Source: CAD feature listing. Evaluate the final solid. Frame: model axes, mm. A direction names the side the tool comes from. Give positions to 0.01 mm unless a question says otherwise; leave off trailing zeros. Loops run counter-clockwise (first coordinate to the right, second up) from the corner with the lowest first, then second, coordinate; pieces in that order, holes last. Notation, with made-up numbers: (-37.75, 72) - (-30.75, 72) arc R30 ccw to (-30.75, 111) - close; hole circle Ø6 at (-22.5, 48). An arc over 180 degrees is marked (long way). Write each question's results on one line, items separated by ' | '. Start each with the question number.
(1) Cut plane D-D on z = -5. Return the cut outline in (x, y).
(2) Cut plane C-C on x = 12.5. Return the cut outline in (y, z), then the cut area to 3 significant figures.
(3) Material intervals for line 1 along Z through (x, y) = (0, 5.1); line 2 along Y through (x, z) = (0, 13), sorted ascending. Write a range as [from, to].
(4) Reachability of faces 5 (the flat face through (4, 5, 10)), 6 (the flat face through (-5, 6, 10)), 7 (the cylindrical face through (-0.27, 0.07, 19.44)) from +Z, -Z, +X, -X, +Y, -Y: full face, straight path, thin tool, end or side. Return the list, or none.
(5) Cut plane B-B on z = 12.5. Return the cut outline in (x, y), then the cut area to 3 significant figures.
(6) Contact query for flat-ended pins moving along their axis: pin 1 (2 mm diameter, centred on x = 2, z = -7, fed in from +Y); pin 2 (1.5 mm diameter, centred on x = -4.5, y = 4, fed in from +Z); pin 3 (1.5 mm diameter, centred on x = -12.5, y = 2, fed in from -Z); pin 4 (17.5 mm diameter, centred on x = -4, z = 0, fed in from +Y). Output: stop coordinate, or through.
(7) Pull-direction query (X, two-part tool) for faces 1 (the cylindrical face through (10, 5.5, -3.2)), 2 (the flat face through (8, 6, -5)), 3 (the cylindrical face through (9.139, 2.958, -14.334)), 4 (the flat face through (0, 2, 0)); classes: pulls with the +X half, pulls with the -X half, needs draft (parallel to the pull), parting line crosses it, or undercut.
from build123d import *

# Parameters (mm, degrees)
SKETCH1_R           = 17
BOSS_EXTRUDE1_DEPTH = 6
SKETCH2_R           = 15
SKETCH2_R_2         = 13.5
CUT_EXTRUDE1_DEPTH  = 1
SKETCH3_R           = 11
SKETCH3_R_2         = 10.5
CUT_EXTRUDE2_DEPTH  = 1
SKETCH4_R           = 9
CUT_EXTRUDE3_DEPTH  = 4
SKETCH8_R           = 1.25
BOSS_EXTRUDE2_DEPTH = 22
SKETCH9_R           = 9
CUT_EXTRUDE5_DEPTH  = 4
SKETCH10_R          = 0.981301711
CUT_EXTRUDE6_DEPTH  = 21


with BuildPart() as part:
    # Sketch1 → Boss-Extrude1 (new body)
    with BuildSketch(Plane(origin=(0, 0, 0), x_dir=(1, 0, 0), z_dir=(0, 1, 0))):
        Circle(SKETCH1_R)
    extrude(amount=BOSS_EXTRUDE1_DEPTH)

    # Sketch2 → Cut-Extrude1 (cut)
    with BuildSketch(Plane(origin=(0, 6, 0), x_dir=(1, 0, 0), z_dir=(0, 1, 0))):
        Circle(SKETCH2_R)
        Circle(SKETCH2_R_2, mode=Mode.SUBTRACT)
    extrude(amount=-CUT_EXTRUDE1_DEPTH, mode=Mode.SUBTRACT)

    # Sketch3 → Cut-Extrude2 (cut)
    with BuildSketch(Plane(origin=(0, 6, 0), x_dir=(1, 0, 0), z_dir=(0, 1, 0))):
        Circle(SKETCH3_R)
        Circle(SKETCH3_R_2, mode=Mode.SUBTRACT)
    extrude(amount=-CUT_EXTRUDE2_DEPTH, mode=Mode.SUBTRACT)

    # Sketch4 → Cut-Extrude3 (cut)
    with BuildSketch(Plane(origin=(0, 6, 0), x_dir=(1, 0, 0), z_dir=(0, 1, 0))):
        Circle(SKETCH4_R)
    extrude(amount=-CUT_EXTRUDE3_DEPTH, mode=Mode.SUBTRACT)

    # Sketch8 → Boss-Extrude2 (add)
    with BuildSketch(Plane.XY):
        with Locations((0, 1.289022222)):
            Circle(SKETCH8_R)
    extrude(amount=BOSS_EXTRUDE2_DEPTH)

    # Sketch9 → Cut-Extrude5 (cut)
    with BuildSketch(Plane(origin=(0, 6, 0), x_dir=(1, 0, 0), z_dir=(0, 1, 0))):
        Circle(SKETCH9_R)
    extrude(amount=-CUT_EXTRUDE5_DEPTH, mode=Mode.SUBTRACT)

    # Sketch10 → Cut-Extrude6 (cut)
    with BuildSketch(Plane.XY.offset(22)):
        with Locations((0, 1.289022222)):
            Circle(SKETCH10_R)
    extrude(amount=-CUT_EXTRUDE6_DEPTH, mode=Mode.SUBTRACT)


solid = part.part
Ans:
1) outline: (-16.25, 0) - (16.25, 0) - (16.25, 6) - (14.14, 6) - (14.14, 5) - (12.54, 5) - (12.54, 6) - (9.8, 6) - (9.8, 5) - (9.23, 5) - (9.23, 6) - (7.48, 6) - (7.48, 2) - (-7.48, 2) - (-7.48, 6) - (-9.23, 6) - (-9.23, 5) - (-9.8, 5) - (-9.8, 6) - (-12.54, 6) - (-12.54, 5) - (-14.14, 5) - (-14.14, 6) - (-16.25, 6) - close
2) outline: (0, -11.52) - (6, -11.52) - (6, -8.29) - (5, -8.29) - (5, -5.1) - (6, -5.1) - (6, 5.1) - (5, 5.1) - (5, 8.29) - (6, 8.29) - (6, 11.52) - (0, 11.52) - close | area: 132 mm^2
3) line 1: [-17, -15], [-13.5, -11], [-10.5, -9], [9, 10.5], [11, 13.5], [15, 17] | line 2: [0, 0.31], [2.27, 6]
4) face 5: +Y | face 6: +Z, -Z, +X, -X, +Y | face 7: +Z
5) outline: (-11.52, 0) - (11.52, 0) - (11.52, 6) - (8.29, 6) - (8.29, 5) - (5.1, 5) - (5.1, 6) - (-5.1, 6) - (-5.1, 5) - (-8.29, 5) - (-8.29, 6) - (-11.52, 6) - close; hole circle Ø1.96 at (0, 1.29) | area: 129 mm^2
6) pin 1: y = 2 | pin 2: z = 16.58 | pin 3: z = -12.29 | pin 4: y = 6
7) face 1: undercut | face 2: needs draft | face 3: parting line crosses it | face 4: undercut
